```python
from build123d import *

# Parameters (mm, degrees)
ESTRUSIONE_ESTRUSIONE1_DEPTH         = 20
TAGLIO_ESTRUSIONE1_REACH             = 37.979
ESTRUSIONE_ESTRUSIONE4_DEPTH         = 0.6
SCHIZZO12_W                          = 2
SCHIZZO12_H                          = 6
TAGLIO_ESTRUSIONE2_DEPTH             = 11
SCHIZZO13_R                          = 3.25
TAGLIO_ESTRUSIONE3_DEPTH             = 27.487921942
TAGLIO_ESTRUSIONE4_REACH             = 34.76
SCHIZZO14_W                          = 18.5
SCHIZZO14_H                          = 9.5
TAGLIO_ESTRUSIONE4_DIRECTION_2_REACH = 34.76
SCHIZZO15_W                          = 1
SCHIZZO15_H                          = 20
ESTRUSIONE_ESTRUSIONE5_DEPTH         = 3


with BuildPart() as part:
    # Schizzo2 → Estrusione-Estrusione1 (new body)
    with BuildSketch(Plane.XY):
        with BuildLine():
            Line((-4, 9.5), (-11, 9.5))
            Line((-11, 9.5), (-11, 23.5))
            Line((-11, 23.5), (-6, 23.5))
            ThreePointArc((-6, 23.5), (-5.292893219, 23.207106781), (-5, 22.5))
            Line((-5, 22.5), (-5, 12.5))
            Line((-5, 12.5), (4, 12.5))
            Line((4, 12.5), (4, 9.5))
            Line((4, 9.5), (4, 6.5))
            Line((4, 6.5), (7.5, 6.5))
            Line((7.5, 6.5), (7.5, 4))
            Line((7.5, 4), (4, 0))
            Line((4, 0), (-4, 0))
            Line((-4, 0), (-7.5, 4))
            Line((-7.5, 4), (-7.5, 6.5))
            Line((-7.5, 6.5), (-4, 6.5))
            Line((-4, 6.5), (-4, 9.5))
        make_face()
    extrude(amount=-ESTRUSIONE_ESTRUSIONE1_DEPTH)

    # Schizzo6 → Taglio-Estrusione1 (cut, up to next)
    with BuildSketch(Plane.ZY.offset(11), mode=Mode.PRIVATE) as taglio_estrusione1_sk1:
        with BuildLine():
            Line((-8.5, 20), (-8.5, 17))
            ThreePointArc((-8.5, 17), (-10, 15.5), (-11.5, 17))
            Line((-11.5, 17), (-11.5, 20))
            ThreePointArc((-11.5, 20), (-10, 21.5), (-8.5, 20))
        make_face()
    taglio_estrusione1_tool1 = extrude(taglio_estrusione1_sk1.sketch, amount=-TAGLIO_ESTRUSIONE1_REACH, mode=Mode.PRIVATE) & part.part
    add(taglio_estrusione1_tool1.solids().sort_by_distance((-11, 18.5, -10))[0], mode=Mode.SUBTRACT)

    # Schizzo11 → Estrusione-Estrusione4 (add)
    with BuildSketch(Plane(origin=(0, 0, -20), x_dir=(-1, 0, 0), z_dir=(0, 0, -1))):
        with BuildLine():
            Line((-1.916666667, 6), (-2.5, 6))
            add(Edge.make_bspline(
                [(-2.5, 6), (-2.484196549, 6.065431756), (-2.453302094, 6.193345487), (-2.388863743, 6.376101829), (-2.318665127, 6.549045511), (-2.234371075, 6.708938219), (-2.142426246, 6.858993324), (-2.037084049, 6.995807413), (-1.923204564, 7.122860063), (-1.797243944, 7.235613218), (-1.665147858, 7.337714716), (-1.525054993, 7.424768393), (-1.379783905, 7.499656106), (-1.228328086, 7.561350822), (-1.070236625, 7.607826795), (-0.906938753, 7.641546577), (-0.738006538, 7.66344436), (-0.623332441, 7.665581492), (-0.565104167, 7.666666667)],
                knots=[0, 0, 0, 0, 1.162005537, 2.271625781, 3.343758855, 4.383309926, 5.390229558, 6.379919256, 7.361854164, 8.333198761, 9.295911338, 10.242430842, 11.177959212, 12.116337295, 13.062827104, 14.020064771, 14.994644689, 16, 16, 16, 16], degree=3))
            add(Edge.make_bspline(
                [(-0.565104167, 7.666666667), (-0.480264789, 7.664105239), (-0.312436625, 7.659038256), (-0.065876681, 7.612768588), (0.171887412, 7.539550485), (0.398253158, 7.438384992), (0.608515961, 7.313608553), (0.795597451, 7.165102613), (0.956961828, 6.995732482), (1.092337101, 6.80865772), (1.198333527, 6.608726059), (1.276493935, 6.402954339), (1.324077057, 6.191830678), (1.330243806, 6.049281445), (1.333333333, 5.977864583)],
                knots=[0, 0, 0, 0, 1.083050992, 2.142477498, 3.193116406, 4.255571735, 5.30263384, 6.308962982, 7.297363603, 8.282367274, 9.249857812, 10.179914175, 11.08814088, 12, 12, 12, 12], degree=3))
            add(Edge.make_bspline(
                [(1.333333333, 5.977864583), (1.331172379, 5.909137679), (1.326943725, 5.774649792), (1.291038272, 5.578309869), (1.230613784, 5.393261183), (1.146912796, 5.218724739), (1.038564203, 5.055807179), (0.907314909, 4.904141953), (0.752238537, 4.763056374), (0.634720509, 4.682234495), (0.57421875, 4.640625)],
                knots=[0, 0, 0, 0, 1.024540389, 2.004866551, 2.965041327, 3.920577974, 4.882998113, 5.874504559, 6.905732034, 8, 8, 8, 8], degree=3))
            add(Edge.make_bspline(
                [(0.57421875, 4.640625), (0.643363437, 4.607236967), (0.780359061, 4.541085617), (0.967095758, 4.411353496), (1.136611813, 4.261563137), (1.231147291, 4.144669639), (1.278645833, 4.0859375)],
                knots=[0, 0, 0, 0, 1.015518401, 2.012035669, 3.001164323, 4, 4, 4, 4], degree=3))
            add(Edge.make_bspline(
                [(1.278645833, 4.0859375), (1.309922612, 4.043115961), (1.37196399, 3.958174116), (1.448544267, 3.821606468), (1.518018337, 3.683525131), (1.572154458, 3.540229091), (1.614077354, 3.393379209), (1.644044271, 3.24272333), (1.662660533, 3.088138431), (1.665326558, 2.983558111), (1.666666667, 2.930989583)],
                knots=[0, 0, 0, 0, 1.025084078, 2.033381695, 3.024893161, 4.013698104, 4.991890475, 5.976764909, 6.982997093, 8, 8, 8, 8], degree=3))
            add(Edge.make_bspline(
                [(1.666666667, 2.930989583), (1.663333999, 2.83997153), (1.656684346, 2.658363755), (1.597248208, 2.390053558), (1.505109333, 2.127777625), (1.374260737, 1.876924352), (1.214792507, 1.64221793), (1.025071762, 1.43221907), (0.807254146, 1.251707377), (0.56432937, 1.100888382), (0.301140417, 0.980326526), (0.019642889, 0.896648418), (-0.276107211, 0.842148704), (-0.478920764, 0.836304519), (-0.58203125, 0.833333333)],
                knots=[0, 0, 0, 0, 0.955779014, 1.907060117, 2.875433937, 3.871313158, 4.872415639, 5.851225146, 6.836215519, 7.83643374, 8.849228613, 9.86973379, 10.916971861, 12, 12, 12, 12], degree=3))
            add(Edge.make_bspline(
                [(-0.58203125, 0.833333333), (-0.651524236, 0.834945729), (-0.78826326, 0.838118387), (-0.9892869, 0.859807218), (-1.181170056, 0.899420085), (-1.364172166, 0.952726223), (-1.538455805, 1.020310887), (-1.703489143, 1.104474184), (-1.860287517, 1.203481259), (-2.007371283, 1.318500779), (-2.144722909, 1.447166124), (-2.268692254, 1.591761428), (-2.381346155, 1.74961375), (-2.479668199, 1.922556569), (-2.568136825, 2.108354904), (-2.640901459, 2.309387829), (-2.704946086, 2.523858156), (-2.73472252, 2.673316816), (-2.75, 2.75)],
                knots=[0, 0, 0, 0, 1.048658725, 2.063410685, 3.046034179, 4.001477787, 4.936774919, 5.862367409, 6.792675028, 7.730719943, 8.675894397, 9.627829632, 10.600096036, 11.597688215, 12.626045268, 13.701542398, 14.82072376, 16, 16, 16, 16], degree=3))
            Line((-2.75, 2.75), (-2.166666667, 2.75))
            add(Edge.make_bspline(
                [(-2.166666667, 2.75), (-2.151469125, 2.699951833), (-2.121908588, 2.602603799), (-2.071590606, 2.462500375), (-2.014263815, 2.33406399), (-1.952765349, 2.216352478), (-1.888176806, 2.108206588), (-1.815906231, 2.012485974), (-1.74130639, 1.924986312), (-1.685073305, 1.875689176), (-1.657552083, 1.8515625)],
                knots=[0, 0, 0, 0, 1.198163088, 2.33053128, 3.407730985, 4.417276592, 5.372219308, 6.28897303, 7.162600585, 8, 8, 8, 8], degree=3))
            add(Edge.make_bspline(
                [(-1.657552083, 1.8515625), (-1.621158441, 1.823504166), (-1.548483496, 1.767474107), (-1.430056781, 1.695971082), (-1.305507707, 1.634014892), (-1.172137598, 1.586688029), (-1.032824452, 1.54661523), (-0.885316488, 1.520391409), (-0.730915085, 1.502399091), (-0.625489239, 1.500811361), (-0.571614583, 1.5)],
                knots=[0, 0, 0, 0, 0.946170439, 1.889420265, 2.845303464, 3.807233317, 4.801018734, 5.828864929, 6.890507805, 8, 8, 8, 8], degree=3))
            add(Edge.make_bspline(
                [(-0.571614583, 1.5), (-0.51078665, 1.501143824), (-0.391842877, 1.503380473), (-0.218283853, 1.523949643), (-0.053170021, 1.553906125), (0.101665412, 1.600173093), (0.24825064, 1.657337532), (0.384530847, 1.729113142), (0.512295044, 1.813324768), (0.629906797, 1.909040348), (0.735662739, 2.013823125), (0.828778978, 2.123418828), (0.907939064, 2.237365369), (0.97179428, 2.356293307), (1.022216731, 2.479710161), (1.056542675, 2.607962273), (1.080409774, 2.740000053), (1.082353483, 2.829753852), (1.083333333, 2.875)],
                knots=[0, 0, 0, 0, 1.217147791, 2.380027433, 3.494444702, 4.572153297, 5.609568379, 6.639424714, 7.649109417, 8.668170816, 9.669597737, 10.625200337, 11.543417969, 12.441394052, 13.322311151, 14.205496177, 15.095365482, 16, 16, 16, 16], degree=3))
            add(Edge.make_bspline(
                [(1.083333333, 2.875), (1.080491345, 2.935563915), (1.074821509, 3.056390388), (1.031534147, 3.234151597), (0.960333399, 3.405423649), (0.860655878, 3.567284402), (0.739318097, 3.71729679), (0.597497555, 3.851143829), (0.43401656, 3.961588284), (0.283551089, 4.037895789), (0.150272941, 4.089964642), (0.036215798, 4.124646719), (-0.091475036, 4.154014937), (-0.231255399, 4.181337727), (-0.384178515, 4.204591659), (-0.5500779, 4.223983603), (-0.728987171, 4.239500107), (-0.852842194, 4.246429284), (-0.916666667, 4.25)],
                knots=[0, 0, 0, 0, 1.07054697, 2.135767047, 3.216561865, 4.33974944, 5.486079747, 6.621378074, 7.775625952, 8.963672916, 9.598146892, 10.304877434, 11.070270905, 11.915000392, 12.823868403, 13.805723172, 14.86925407, 16, 16, 16, 16], degree=3))
            Line((-0.916666667, 4.25), (-0.916666667, 4.916666667))
            add(Edge.make_bspline(
                [(-0.916666667, 4.916666667), (-0.836250216, 4.918031302), (-0.678734144, 4.920704288), (-0.448644721, 4.95303345), (-0.228622855, 4.997754616), (-0.02354462, 5.066255688), (0.163374419, 5.145816239), (0.325539394, 5.238398914), (0.460678382, 5.34131202), (0.568134658, 5.456144008), (0.648974654, 5.579300525), (0.708081563, 5.707660032), (0.742996455, 5.842347574), (0.747657265, 5.934266243), (0.75, 5.98046875)],
                knots=[0, 0, 0, 0, 1.321986639, 2.589447074, 3.816329219, 5.01088745, 6.139805852, 7.153945165, 8.075214402, 8.924034688, 9.728124013, 10.488707548, 11.240355623, 12, 12, 12, 12], degree=3))
            add(Edge.make_bspline(
                [(0.75, 5.98046875), (0.74923038, 6.014413134), (0.747699256, 6.081943876), (0.728390026, 6.180604717), (0.69937395, 6.276249331), (0.659483024, 6.368470979), (0.606089798, 6.456630059), (0.542192966, 6.541478178), (0.466109351, 6.622530911), (0.37892495, 6.698080076), (0.285303026, 6.770080088), (0.182696301, 6.831205413), (0.074198534, 6.883474814), (-0.040310397, 6.926578176), (-0.161202096, 6.959002568), (-0.28790856, 6.982283416), (-0.420671401, 6.996839061), (-0.511247475, 6.99893469), (-0.557291667, 7)],
                knots=[0, 0, 0, 0, 0.884392785, 1.759457502, 2.611959086, 3.489218968, 4.37281399, 5.2945488, 6.255912374, 7.266815255, 8.301784654, 9.332968512, 10.37626691, 11.440494194, 12.520033166, 13.637162961, 14.798855837, 16, 16, 16, 16], degree=3))
            add(Edge.make_bspline(
                [(-0.557291667, 7), (-0.631301907, 6.997416042), (-0.775861121, 6.992368971), (-0.984260252, 6.948163375), (-1.177996158, 6.877632648), (-1.326082253, 6.793442755), (-1.435435605, 6.710334806), (-1.51357849, 6.637753232), (-1.590316581, 6.557092273), (-1.660601409, 6.463383862), (-1.731681652, 6.362974109), (-1.79639298, 6.2507587), (-1.859275266, 6.129664825), (-1.897165715, 6.044058647), (-1.916666667, 6)],
                knots=[0, 0, 0, 0, 1.472543308, 2.876219568, 4.221790263, 5.565193594, 6.249813518, 6.953379497, 7.687249741, 8.463570142, 9.283606569, 10.136032583, 11.040678096, 12, 12, 12, 12], degree=3))
        make_face()
    extrude(amount=ESTRUSIONE_ESTRUSIONE4_DEPTH)

    # Schizzo12 → Taglio-Estrusione2 (cut)
    with BuildSketch(Plane(origin=(0, 23.5, 0), x_dir=(1, 0, 0), z_dir=(0, 1, 0))):
        with Locations((-8.5, 10)):
            Rectangle(SCHIZZO12_W, SCHIZZO12_H)
    extrude(amount=-TAGLIO_ESTRUSIONE2_DEPTH, mode=Mode.SUBTRACT)

    # Schizzo13 → Taglio-Estrusione3 (cut, through all)
    with BuildSketch(Plane(origin=(0, 12.5, 0), x_dir=(1, 0, 0), z_dir=(0, 1, 0))):
        with Locations(Location((0, 10, 0), (0, 0, 180))):
            Circle(SCHIZZO13_R)
    extrude(amount=-TAGLIO_ESTRUSIONE3_DEPTH, mode=Mode.SUBTRACT)

    # Schizzo14 → Taglio-Estrusione4 (cut, up to next)
    with BuildSketch(Plane(origin=(0, 0, -20), x_dir=(-1, 0, 0), z_dir=(0, 0, -1)), mode=Mode.PRIVATE) as taglio_estrusione4_sk1:
        with Locations((1.75, 4.75)):
            Rectangle(SCHIZZO14_W, SCHIZZO14_H)
    taglio_estrusione4_tool1 = extrude(taglio_estrusione4_sk1.sketch, amount=-TAGLIO_ESTRUSIONE4_REACH, mode=Mode.PRIVATE) & part.part
    add(taglio_estrusione4_tool1.solids().sort_by_distance((-1.75, 4.75, -20))[0], mode=Mode.SUBTRACT)

    # Schizzo14 → Taglio-Estrusione4 direction 2 (cut, up to next)
    with BuildSketch(Plane(origin=(0, 0, -20), x_dir=(-1, 0, 0), z_dir=(0, 0, -1)), mode=Mode.PRIVATE) as taglio_estrusione4_direction_2_sk1:
        with Locations((1.75, 4.75)):
            Rectangle(SCHIZZO14_W, SCHIZZO14_H)
    taglio_estrusione4_direction_2_tool1 = extrude(taglio_estrusione4_direction_2_sk1.sketch, amount=TAGLIO_ESTRUSIONE4_DIRECTION_2_REACH, mode=Mode.PRIVATE) & part.part
    add(taglio_estrusione4_direction_2_tool1.solids().sort_by_distance((-1.75, 4.75, -20))[0], mode=Mode.SUBTRACT)

    # Schizzo15 → Estrusione-Estrusione5 (add, through all)
    with BuildSketch(Plane(origin=(0, 12.5, 0), x_dir=(1, 0, 0), z_dir=(0, 1, 0))):
        with Locations((4.5, 10)):
            Rectangle(SCHIZZO15_W, SCHIZZO15_H)
    extrude(amount=-ESTRUSIONE_ESTRUSIONE5_DEPTH)


solid = part.part
```
The listing builds one solid part. Answer for the finished solid, in the listing's coordinates (mm). A direction names the side the tool comes from. Coordinates: 2 decimals unless noted, no trailing zeros. Loops run counter-clockwise (first coordinate to the right, second up) from the corner with the lowest first, then second, coordinate; pieces in that order, holes last. Notation, with made-up numbers: (-22, 42) - (32, 42) arc R16 ccw to (32, 58) - close; hole circle Ø3 at (-0.5, 43). An arc over 180 degrees is marked (long way). Write item = value, one per line.
1) Section C-C (x = 0) is taken. Determine the outline of the cut face in (y, z), plus the area to 3 significant figures.
Responses:
outline = (9.5, -20) - (12.5, -20) - (12.5, -13.25) - (9.5, -13.25) - close; (9.5, -6.75) - (12.5, -6.75) - (12.5, 0) - (9.5, 0) - close
area = 40.5 mm^2
2) Section A-A (z = -10) is taken. Determine the outline of the cut face in (x, y), plus the area to 3 significant figures.
Responses:
outline = (-11, 9.5) - (-3.25, 9.5) - (-3.25, 12.5) - (-5, 12.5) - (-5, 15.5) - (-7.5, 15.5) - (-7.5, 12.5) - (-9.5, 12.5) - (-9.5, 15.5) - (-11, 15.5) - close; (-11, 21.5) - (-9.5, 21.5) - (-9.5, 23.5) - (-11, 23.5) - close; (-7.5, 21.5) - (-5, 21.5) - (-5, 22.5) arc R1 ccw to (-6, 23.5) - (-7.5, 23.5) - close; (3.25, 9.5) - (5, 9.5) - (5, 12.5) - (3.25, 12.5) - close
area = 48.3 mm^2
3) Which of the six approach directions +Z, -Z, +X, -X, +Y, -Y give full straight-line access (tool end or side, diameter ignored) to faces 1 (the face through (-3.4, 12.5, -10.1)), 2 (the face through (-10.3, 21.5, -10)), 3 (the face through (-9.5, 18, -12))?
Responses:
face_1 = +Z, -Z, +X, +Y
face_2 = +X, -X
face_3 = +Y
4) Find the intervals of material crossed by line 1 along Z through (x, y) = (0, 11.25); line 2 along X through (y, z) = (14.5, -7.75); line 3 along Y through (x, z) = (-1.75, -6), in increasing order.
Responses:
line_1 = -20 to -13.25, -6.75 to 0
line_2 = -11 to -9.5, -7.5 to -5
line_3 = 9.5 to 12.5
5) Section B-B (y = 13.25) is taken. Determine the outline of the cut face in (x, z), plus the area to 3 significant figures.
Responses:
outline = (-11, -20) - (-5, -20) - (-5, 0) - (-11, 0) - close; hole (-9.5, -13) - (-7.5, -13) - (-7.5, -7) - (-9.5, -7) - close
area = 108 mm^2
6) Determine the mould class of faces 4 (the face through (-10, 23.5, -10)), 5 (the face through (-6.3, 15.5, -10)), 6 (the face through (-7, 15, -20)) for opening direction Z: pulls with the +Z half, pulls with the -Z half, needs draft (parallel to the pull), parting line crosses it, or undercut.
Responses:
face_4 = needs draft
face_5 = undercut
face_6 = pulls with the -Z half
7) Each of these flat-tipped pins is pushed along its axis until it touches: P1, Ø1.6, axis at x = -10.5, y = 19, coming from the +Z side; P2, Ø7.5, axis at x = 0, z = -10, coming from the +Y side; P3, Ø2, axis at y = 14.5, z = -6, coming from the +X side; P4, Ø4, axis at x = -3.5, z = -4.5, coming from the +Y side. Where does it stop, or does it pass through?
Responses:
P1 = 0
P2 = 12.5
P3 = -5
P4 = 23.37
8) Section D-D (y = 20.25) is taken. Determine the outline of the cut face in (x, z), plus the area to 3 significant figures.
Responses:
outline = (-11, -20) - (-5, -20) - (-5, -11.48) - (-7.5, -11.48) - (-7.5, -13) - (-9.5, -13) - (-9.5, -11.48) - (-11, -11.48) - close; (-11, -8.52) - (-9.5, -8.52) - (-9.5, -7) - (-7.5, -7) - (-7.5, -8.52) - (-5, -8.52) - (-5, 0) - (-11, 0) - close
area = 96.2 mm^2
